from build123d import *

# Parameters (mm, degrees)
F0_R     = 11.15
F1_DEPTH = 6.585
F3_DEPTH = 25


with BuildPart() as f1:
    # F0 (on Top) → F1 (new body)
    with BuildSketch(Plane.XY):
        with BuildLine():
            Line((-9.824942, -28.391755), (0, -45.409054))
            Line((0, -45.409054), (11.093962, -26.193747))
            Line((11.093962, -26.193747), (10.476884, -22.719322))
            Line((10.476884, -22.719322), (9.30388, -16.114792))
            ThreePointArc((9.30388, -16.114792), (14.198421, -8.08372), (18.898248, 0.062829))
            Line((18.898248, 0.062829), (24.486244, 3.027224))
            Line((24.486244, 3.027224), (29.500452, 5.687228))
            Line((29.500452, 5.687228), (39.325394, 22.704527))
            Line((39.325394, 22.704527), (17.137469, 22.704527))
            Line((17.137469, 22.704527), (9.30388, 16.114792))
            ThreePointArc((9.30388, 16.114792), (-0.098503, 16.338053), (-9.503536, 16.334949))
            Line((-9.503536, 16.334949), (-19.67551, 22.704527))
            Line((-19.67551, 22.704527), (-39.325394, 22.704527))
            Line((-39.325394, 22.704527), (-28.231432, 3.48922))
            Line((-28.231432, 3.48922), (-18.607759, 0))
            ThreePointArc((-18.607759, 0), (-14.099918, -8.254333), (-9.394713, -16.397778))
            Line((-9.394713, -16.397778), (-9.824942, -28.391755))
        make_face()
        Circle(F0_R, mode=Mode.SUBTRACT)
    extrude(amount=F1_DEPTH)

    # F2 (on face) → F3 (cut)
    with BuildSketch(Plane(origin=(0, 0, 0), x_dir=(1, 0, 0), z_dir=(0, 0, -1))):
        Polygon((-2.199187, 29.137347), (-2.199187, 18.615887), (1.608272, 18.904826), (1.608272, 29.137347), align=None)
        Polygon((-24.134089, -16.473225), (-15.022237, -11.212495), (-17.176195, -8.059608), (-26.037819, -13.175869), align=None)
        Polygon((26.333276, -12.664122), (17.221424, -7.403392), (15.567923, -10.845217), (24.429547, -15.961478), align=None)
    extrude(amount=-F3_DEPTH, mode=Mode.SUBTRACT)


solid = f1.part
Input: part model. Units: mm. Frame: model coordinates. A direction names the side the tool comes from. Round coordinates to 2 decimals unless told otherwise and drop trailing zeros. Loops run counter-clockwise (first coordinate to the right, second up) from the corner with the lowest first, then second, coordinate; pieces in that order, holes last. Notation, with made-up numbers: M -9.5,77 L 32.5,77 A28 ccw 32.5,101 Z; hole C 60.25,2.5 d6. An arc over 180 degrees is marked long. Answer as CSV lines item,"result". Start each with the question number.
(1) Section C-C, the plane y = -34.5. Output: boundary loops of the cut face in (x, z) (3 decimals).
(2) Section A-A, the plane z = 3.75. State how many separate pieces and enclosed holes the cut face has, plus the area to 3 significant figures.
(3) Section B-B, the plane x = -5. Output: boundary loops of the cut face in (y, z) (3 decimals), plus the area to 3 significant figures.
(4) Line query: line 1 (X direction, y = 14, z = 5.75); line 2 (Y direction, x = -20, z = 5); line 3 (X direction, y = 4, z = 2.5). Output: solid intervals per line, ascending. Write a range as [from, to].
(5) Section D-D, the plane y = -13. Output: boundary loops of the cut face in (x, z) (3 decimals).
(6) Draft query along X for faces 4 (the cylindrical face through (14.13, -8.2, 3.25)), 5 (the flat face through (-12, -1, 6.585)), 6 (the flat face through (0, -29.137, 3)), 7 (the cylindrical face through (-14.164, -8.14, 3.246)). Return one class per face: released by +X, released by -X, zero draft, split by the parting line, or undercut.
(7) Reachability of faces 1 (the flat face through (21.84, 10.07, 3.25)), 2 (the flat face through (-23.49, 1.77, 3.25)), 3 (the cylindrical face through (0.033, 16.336, 3.246)) from +Z, -Z, +X, -X, +Y, -Y: full face, straight path, thin tool, end or side. Return the list, or none.
(8) First-contact query: pin 1 (1 mm diameter, centred on x = -17.5, z = 2, fed in from +Y); pin 2 (1 mm diameter, centred on y = 16, z = 0.5, fed in from -X); pin 3 (1 mm diameter, centred on y = -28, z = 1, fed in from -X). Flat tips, straight axial feed; report the tip coordinate or a pass-through.
Values found:
1,outline,"M -6.298,0 L 6.298,0 L 6.298,6.585 L -6.298,6.585 Z"
2,separate pieces,"1"
2,enclosed holes,"4"
2,area,"1,630 mm²"
3,outline,"M -36.749,0 L -9.966,0 L -9.966,6.585 L -36.749,6.585 Z; M 9.966,0 L 16.365,0 L 16.365,6.585 L 9.966,6.585 Z"
3,area,"218 mm²"
4,line 1,"x = [-34.3, -25.56], [-19.85, 21.03], [25.56, 34.3]"
4,line 2,"y = [0.5, 9.69], [14.09, 22.7]"
4,line 3,"x = [-28.53, -10.41], [10.41, 26.32]"
5,outline,"M -11.39,0 L 11.234,0 L 11.234,6.585 L -11.39,6.585 Z"
6,face 4,"released by +X"
6,face 5,"zero draft"
6,face 6,"undercut"
6,face 7,"released by -X"
7,face 1,"+Z, -Z"
7,face 2,"+Z, -Z, -X, -Y"
7,face 3,"+Z, -Z, +Y"
8,pin 1,"stops at y = 21.66"
8,pin 2,"stops at x = -35.74"
8,pin 3,"stops at x = -9.82"
